Study the drawing (mm; zero at the part's minimum x, y, z) and answer. A direction names the side the tool comes from. Coordinates: 2 decimals unless noted, no trailing zeros. Order: outer loops, then holes, each group sorted by start corner. A loop starts at its lowest first (then second) coordinate and runs counter-clockwise, first axis right, second up.
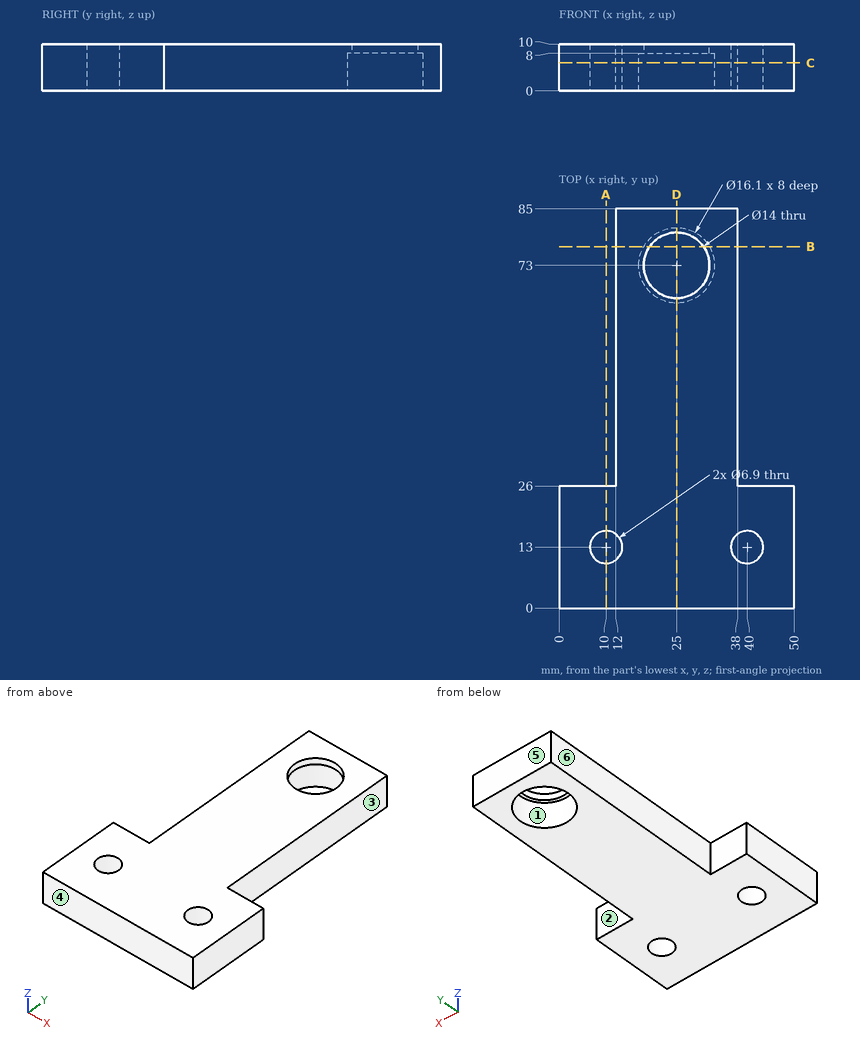
(1) Find the intervals of material crossed by probe 1 along Y at (x, z) = (40, 6.5); probe 2 along Y at (x, z) = (25, 8.7); probe 3 along X at (y, z) = (73, 8.75), in increasing order.
(2) Find section D-D on x = 25. Determine the outline of the cut face in (y, z).
(3) Given pin 1 Ø5 at (y, z) = (70, 6.5) entering from -X; pin 2 Ø6 at (y, z) = (76.5, 5.5) entering from +X; pin 3 Ø17.5 at (x, y) = (21.5, 76) entering from -Z, each flat-ended and moving along its own axis, determine where each tip first touches the part or whether it passes through.
(4) Find section A-A on x = 10. Determine the outline of the cut face in (y, z), then the cut area to 3 significant figures.
(5) Find section C-C on z = 6. Determine the outline of the cut face in (x, y), then the cut area to 3 significant figures.
(6) A tool of negligible diameter and unlimited length cuts with its end or side. For the marked faces 5 and 6, from which of +Z, -Z, +X, -X, +Y, -Y can it reach the whole face along a straight path? Write none if from no direction.
(7) Find section B-B on y = 77. Determine the outline of the cut face in (x, z), then the cut area to 3 significant figures.
(8) The mould has two halves that part along Y. Classify the marked faces 1, 2, 3 and 4: pulls with the +Y half, pulls with the -Y half, needs draft (parallel to the pull), parting line crosses it, or undercut.
Resolved:
1. probe 1: y = 0 to 9.55, 16.45 to 26
1. probe 2: y = 0 to 66, 80 to 85
1. probe 3: x = 12 to 18, 32 to 38
2. outline: (0, 0) - (64.95, 0) - (64.95, 8) - (66, 8) - (66, 10) - (0, 10) - close; (80, 8) - (81.05, 8) - (81.05, 0) - (85, 0) - (85, 10) - (80, 10) - close
3. pin 1: stops at x = 12
3. pin 2: stops at x = 38
3. pin 3: stops at z = 0
4. outline: (0, 0) - (9.55, 0) - (9.55, 10) - (0, 10) - close; (16.45, 0) - (26, 0) - (26, 10) - (16.45, 10) - close
4. area: 191 mm2
5. outline: (0, 0) - (50, 0) - (50, 26) - (38, 26) - (38, 85) - (12, 85) - (12, 26) - (0, 26) - close; hole circle Ø6.9 at (10, 13); hole circle Ø16.1 at (25, 73); hole circle Ø6.9 at (40, 13)
5. area: 2,560 mm2
6. face 5: +Z, -Z, +X, -X, +Y
6. face 6: +Z, -Z, -X, +Y
7. outline: (12, 0) - (18.01, 0) - (18.01, 8) - (19.26, 8) - (19.26, 10) - (12, 10) - close; (30.74, 8) - (31.99, 8) - (31.99, 0) - (38, 0) - (38, 10) - (30.74, 10) - close
7. area: 125 mm2
8. face 1: undercut
8. face 2: pulls with the +Y half
8. face 3: needs draft
8. face 4: pulls with the -Y half
